from build123d import *

# Parameters (mm, degrees)
SKETCH_1_W      = 10
SKETCH_1_H      = 10
SKETCH_1_W_2    = 24
EXTRUDE_1_DEPTH = 300


with BuildPart() as part:
    # Sketch 1 → Extrude 1 (new body)
    with BuildSketch(Plane(origin=(0, 0, 0), x_dir=(1, 0, 0), z_dir=(0, 1, 0))):
        with Locations((0, 10)):
            Rectangle(SKETCH_1_W, SKETCH_1_H)
        with Locations((17, 0)):
            Rectangle(SKETCH_1_W_2, SKETCH_1_H)
        with Locations((-17, 0)):
            Rectangle(SKETCH_1_W_2, SKETCH_1_H)
        Rectangle(SKETCH_1_W, SKETCH_1_H)
        with Locations((0, -10)):
            Rectangle(SKETCH_1_W, SKETCH_1_H)
        Polygon((-40, -15), (-40, 15), (-5, 15), (5, 15), (40, 15), (50, 15), (50, 25), (-50, 25), (-50, -25), (50, -25), (50, -15), (40, -15), (5, -15), (-5, -15), align=None)
    extrude(amount=EXTRUDE_1_DEPTH)


solid = part.part
Design review of the part built by this model. Coordinates are the model's own, in mm. A direction names the side the tool comes from. Round coordinates to 2 decimals unless told otherwise and drop trailing zeros. Write each loop counter-clockwise with the first axis right and the second up, starting at its lowest first coordinate (ties: lowest second). Pieces come first, ordered by that corner, then holes. Notation, with made-up numbers: M 60,-7 L 108,-7 A22 ccw 108,25 Z; hole C 63,13.25 d1. An arc over 180 degrees is marked long. One line per item, written item: value. Start each with the question number.
1. Take a section at D-D on x = -9. State the section outline as (y, z) points.
2. Take a section at B-B on y = 83. State the section outline as (x, z) points.
3. Draft analysis for pull direction Z (two halves, no side actions). For faces 4 (the face through (1, 148, -25)), 5 (the face through (27, 148, -15)), 6 (the face through (-1, 0, 0)), state which applies: pulls with the +Z half, pulls with the -Z half, needs draft (parallel to the pull), parting line crosses it, or undercut.
4. To check wall thickness, follow probe 1 along Z at (x, y) = (-22.5, 145.5); probe 2 along X at (y, z) = (100, -0.5); probe 3 along X at (y, z) = (233.5, -6). State the ranges of each line that lie inside material, in increasing order. Write a range as from..to.
5. Take a section at A-A on z = 0.5. State the section outline as (x, y) points.
6. For faces 1 (the face through (-29, 148, 0)), 2 (the face through (-50, 148, 0)), 3 (the face through (17, 148, -5)), list the 3-axis set-ups (+Z, -Z, +X, -X, +Y, -Y) from which the entire face can be reached by the end or side of a thin tool; tool diameter is ignored.
7. Clearance check with a flat-ended pin moving along its axis: P1, Ø11, axis at y = 98.5, z = 2, coming from the +X side. State where the tip first meets the part, or that it passes through.
8. Take a section at C-C on x = 34.5. State the section outline as (y, z) points.
Computed:
1. outline: M 0,-25 L 300,-25 L 300,-15 L 0,-15 Z; M 0,-5 L 300,-5 L 300,5 L 0,5 Z; M 0,15 L 300,15 L 300,25 L 0,25 Z
2. outline: M -50,-25 L 50,-25 L 50,-15 L 5,-15 L 5,-5 L 29,-5 L 29,5 L 5,5 L 5,15 L 50,15 L 50,25 L -50,25 Z; hole M -40,-15 L -5,-15 L -5,-5 L -29,-5 L -29,5 L -5,5 L -5,15 L -40,15 Z
3. face 4: pulls with the -Z half
3. face 5: undercut
3. face 6: needs draft
4. probe 1: z = -25..-15, -5..5, 15..25
4. probe 2: x = -50..-40, -29..29
4. probe 3: x = -50..-40, -5..5
5. outline: M -50,0 L -40,0 L -40,300 L -50,300 Z; M -29,0 L 29,0 L 29,300 L -29,300 Z
6. face 1: +Y, -Y
6. face 2: +Z, -Z, -X, +Y, -Y
6. face 3: +X, +Y, -Y
7. P1: stops at x = 29
8. outline: M 0,-25 L 300,-25 L 300,-15 L 0,-15 Z; M 0,15 L 300,15 L 300,25 L 0,25 Z
